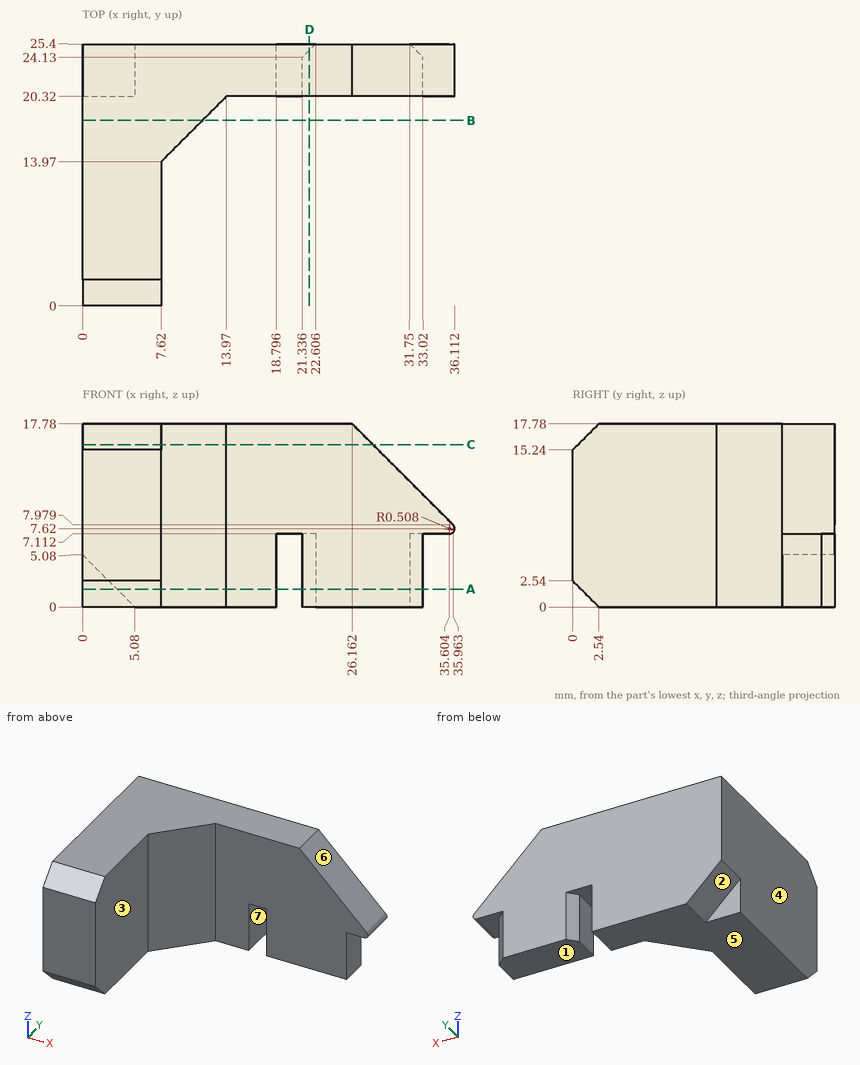
Drawing for the job (mm, zero at the part's lowest x, y, z). A direction names the side the tool comes from. Give positions to 0.01 mm unless a question says otherwise; leave off trailing zeros. Write each loop counter-clockwise with the first axis right and the second up, starting at its lowest first coordinate (ties: lowest second). Pieces come first, ordered by that corner, then holes. Notation, with made-up numbers: (25.5, -4.75) -> (55.5, -4.75) arc R36 cw to (55.5, 34.25) -> close; hole circle Ø11 at (32, -14.75). An arc over 180 degrees is marked (long way). Put each result on its own line as item: value. Start each with the question number.
Item 1: Cut at A-A (z = 1.75). List the corners of the cut face in (x, y), then the cut area to 3 significant figures.
Item 2: Pull direction X, two halves, no side cores. Call the marked faces 4, 5, 6 and 7: pulls with the +X half, pulls with the -X half, needs draft (parallel to the pull), parting line crosses it, or undercut.
Item 3: Which spindle directions (+Z, -Z, +X, -X, +Y, -Y) get a long thin tool onto all of the face, cutting with end or side? Do the marked faces 1, 2 and 3. Say none if no direction does.
Item 4: Pin check, flat tips, straight feed: pin 1 Ø2.5 at (x, z) = (1.5, 1.5) entering from +Y; pin 2 Ø3 at (y, z) = (22.5, 2) entering from -X; pin 3 Ø2 at (x, z) = (19, 4.5) entering from -Y; pin 4 Ø3 at (x, y) = (21, 22) entering from -Z. Stop position of each tip, or through.
Item 5: Wall check: L1, parallel to Y at x = 19, z = 15.25; L2, parallel to X at y = 3, z = 9; L3, parallel to X at y = 22.5, z = 14.5. Give the ranges that are in metal, low to high. Write a range as [from, to].
Item 6: Cut at D-D (x = 22). List the corners of the cut face in (y, z).
Item 7: Cut at C-C (z = 15.75). List the corners of the cut face in (x, y), then the cut area to 3 significant figures.
Item 8: Cut at B-B (y = 18). List the corners of the cut face in (x, z).
Answer list:
1. outline: (0, 0.79) -> (7.62, 0.79) -> (7.62, 13.97) -> (13.97, 20.32) -> (18.8, 20.32) -> (18.8, 25.4) -> (3.33, 25.4) -> (3.33, 20.32) -> (0, 20.32) -> close; (21.34, 20.32) -> (33.02, 20.32) -> (33.02, 24.13) -> (31.75, 25.4) -> (22.61, 25.4) -> (21.34, 24.13) -> close
1. area: 305 mm2
2. face 4: pulls with the -X half
2. face 5: needs draft
2. face 6: pulls with the +X half
2. face 7: undercut
3. face 1: -Z, +X, -X, +Y, -Y
3. face 2: -Z, -X, +Y
3. face 3: +Z, -Z, +X, -Y
4. pin 1: stops at y = 20.32
4. pin 2: stops at x = 1.58
4. pin 3: stops at y = 20.32
4. pin 4: stops at z = 0
5. L1: y = [20.32, 25.4]
5. L2: x = [0, 7.62]
5. L3: x = [0, 29.44]
6. outline: (20.32, 0) -> (24.79, 0) -> (24.79, 7.11) -> (25.4, 7.11) -> (25.4, 17.78) -> (20.32, 17.78) -> close
7. outline: (0, 0.51) -> (7.62, 0.51) -> (7.62, 13.97) -> (13.97, 20.32) -> (28.19, 20.32) -> (28.19, 25.4) -> (0, 25.4) -> close
7. area: 314 mm2
8. outline: (0, 0) -> (11.65, 0) -> (11.65, 17.78) -> (0, 17.78) -> close
